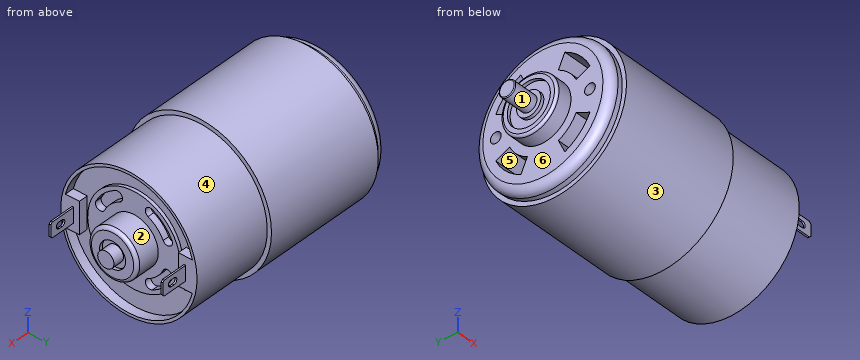
```python
from build123d import *

# Parameters (mm, degrees)
SKETCH1_W                      = 38
SKETCH1_H                      = 22.3
SKETCH2_R                      = 21
BOSS_EXTRUDE1_DEPTH            = 25
SKETCH3_W                      = 4.6
SKETCH3_H                      = 0.5
BOSS_EXTRUDE2_DEPTH            = 8.15
CUT_EXTRUDE1_DEPTH             = 40.8
SKETCH5_W                      = 4.6
SKETCH5_H                      = 0.5
BOSS_EXTRUDE3_DEPTH            = 8.15
CUT_EXTRUDE2_REACH             = 41.8
CUT_EXTRUDE3_DEPTH             = 2.8
SKETCH8_R                      = 14.25
BOSS_EXTRUDE4_DEPTH            = 1
CUT_EXTRUDE4_DEPTH             = 2
CUT_EXTRUDE5_DEPTH             = 2
CUT_EXTRUDE6_DEPTH             = 2
CUT_EXTRUDE7_DEPTH             = 2
SKETCH13_R                     = 21
BOSS_EXTRUDE5_DEPTH            = 4
CUT_EXTRUDE8_DEPTH             = 10
CUT_EXTRUDE9_DEPTH             = 10
CUT_EXTRUDE10_DEPTH            = 10
CUT_EXTRUDE11_DEPTH            = 10
SKETCH18_R                     = 7.5
BOSS_EXTRUDE6_DEPTH            = 7.6
F_8_0_8_DIAMETER_HOLE1_D       = 8
F_8_0_8_DIAMETER_HOLE1_DEPTH   = 1
SKETCH21_R                     = 8.65
BOSS_EXTRUDE7_DEPTH            = 5
M12_CLEARANCE_HOLE1_D          = 13.25
M12_CLEARANCE_HOLE1_DEPTH      = 1
SKETCH25_W                     = 3.4
SKETCH25_H                     = 2.5
F_2_5_2_5_DIAMETER_HOLE1_D     = 2.5
F_2_5_2_5_DIAMETER_HOLE1_DEPTH = 0.1
F_3_3_3_3_DIAMETER_HOLE1_D     = 3.3
F_3_3_3_3_DIAMETER_HOLE1_DEPTH = 11.5
F_3_3_3_3_DIAMETER_HOLE1_TIP   = 0.991420021
CHAMFER1_SIZE                  = 0.5
FILLET1_R                      = 0.25
FILLET2_R                      = 0.75
FILLET3_R                      = 1
FILLET4_R                      = 2.5


with BuildPart() as part:
    # Sketch1 → Revolve1 (revolve)
    with BuildSketch(Plane.XY):
        with Locations((23, 11.15)):
            Rectangle(SKETCH1_W, SKETCH1_H)
    revolve(axis=Axis((4, 0, 0), (1, 0, 0)))

    # Sketch2 → Boss-Extrude1 (add)
    with BuildSketch(Plane(origin=(42, 0, 0), x_dir=(0, 0, -1), z_dir=(1, 0, 0))):
        Circle(SKETCH2_R)
    extrude(amount=BOSS_EXTRUDE1_DEPTH)

    # Sketch3 → Boss-Extrude2 (add)
    with BuildSketch(Plane(origin=(67, 0, 0), x_dir=(0, 0, -1), z_dir=(1, 0, 0))):
        with Locations((0, 17.25)):
            Rectangle(SKETCH3_W, SKETCH3_H)
    extrude(amount=BOSS_EXTRUDE2_DEPTH)

    # Sketch4 → Cut-Extrude1 (cut, through all)
    with BuildSketch(Plane(origin=(0, 17.5, 0), x_dir=(-1, 0, 0), z_dir=(0, 1, 0))):
        with BuildLine():
            Line((-72.15, -1), (-71.15, -1))
            ThreePointArc((-71.15, -1), (-70.15, 0), (-71.15, 1))
            Line((-71.15, 1), (-72.15, 1))
            ThreePointArc((-72.15, 1), (-73.15, 0), (-72.15, -1))
        make_face()
    extrude(amount=-CUT_EXTRUDE1_DEPTH, mode=Mode.SUBTRACT)

    # Sketch5 → Boss-Extrude3 (add)
    with BuildSketch(Plane(origin=(67, 0, 0), x_dir=(0, 0, -1), z_dir=(1, 0, 0))):
        with Locations((0, -17.25)):
            Rectangle(SKETCH5_W, SKETCH5_H)
    extrude(amount=BOSS_EXTRUDE3_DEPTH)

    # Sketch6 → Cut-Extrude2 (cut, up to next)
    with BuildSketch(Plane.XZ.offset(17.5), mode=Mode.PRIVATE) as cut_extrude2_sk1:
        with BuildLine():
            Line((72.15, 1), (71.15, 1))
            ThreePointArc((71.15, 1), (70.15, 0), (71.15, -1))
            Line((71.15, -1), (72.15, -1))
            ThreePointArc((72.15, -1), (73.15, 0), (72.15, 1))
        make_face()
    cut_extrude2_tool1 = extrude(cut_extrude2_sk1.sketch, amount=-CUT_EXTRUDE2_REACH, mode=Mode.PRIVATE) & part.part
    add(cut_extrude2_tool1.solids().sort_by_distance((71.65, -17.5, 0))[0], mode=Mode.SUBTRACT)

    # Sketch7 → Cut-Extrude3 (cut)
    with BuildSketch(Plane(origin=(67, 0, 0), x_dir=(0, 0, -1), z_dir=(1, 0, 0))):
        with BuildLine():
            Line((4.875, 19.551390616), (4.875, 15.25))
            Line((4.875, 15.25), (-4.875, 15.25))
            Line((-4.875, 15.25), (-4.875, 19.551390616))
            ThreePointArc((-4.875, 19.551390616), (-20.15, 0), (-4.875, -19.551390616))
            Line((-4.875, -19.551390616), (-4.875, -15.25))
            Line((-4.875, -15.25), (4.875, -15.25))
            Line((4.875, -15.25), (4.875, -19.551390616))
            ThreePointArc((4.875, -19.551390616), (20.15, 0), (4.875, 19.551390616))
        make_face()
    extrude(amount=-CUT_EXTRUDE3_DEPTH, mode=Mode.SUBTRACT)

    # Sketch8 → Boss-Extrude4 (add)
    with BuildSketch(Plane(origin=(64.2, 0, 0), x_dir=(0, 0, -1), z_dir=(1, 0, 0))):
        Circle(SKETCH8_R)
    extrude(amount=BOSS_EXTRUDE4_DEPTH)

    # Sketch9 → Cut-Extrude4 (cut)
    with BuildSketch(Plane(origin=(65.2, 0, 0), x_dir=(0, 0, -1), z_dir=(1, 0, 0))):
        with BuildLine():
            ThreePointArc((-5.652173913, 11.706960752), (-9.192388155, 9.192388155), (-11.706960752, 5.652173913))
            ThreePointArc((-11.706960752, 5.652173913), (-11.008331502, 3.649196836), (-9.005354425, 4.347826087))
            ThreePointArc((-9.005354425, 4.347826087), (-7.071067812, 7.071067812), (-4.347826087, 9.005354425))
            ThreePointArc((-4.347826087, 9.005354425), (-3.649196836, 11.008331502), (-5.652173913, 11.706960752))
        make_face()
    extrude(amount=-CUT_EXTRUDE4_DEPTH, mode=Mode.SUBTRACT)

    # Sketch10 → Cut-Extrude5 (cut)
    with BuildSketch(Plane(origin=(65.2, 0, 0), x_dir=(0, 0, -1), z_dir=(1, 0, 0))):
        with BuildLine():
            ThreePointArc((11.706960752, 5.652173913), (9.192388155, 9.192388155), (5.652173913, 11.706960752))
            ThreePointArc((5.652173913, 11.706960752), (3.649196836, 11.008331502), (4.347826087, 9.005354425))
            ThreePointArc((4.347826087, 9.005354425), (7.071067812, 7.071067812), (9.005354425, 4.347826087))
            ThreePointArc((9.005354425, 4.347826087), (11.008331502, 3.649196836), (11.706960752, 5.652173913))
        make_face()
    extrude(amount=-CUT_EXTRUDE5_DEPTH, mode=Mode.SUBTRACT)

    # Sketch11 → Cut-Extrude6 (cut)
    with BuildSketch(Plane(origin=(65.2, 0, 0), x_dir=(0, 0, -1), z_dir=(1, 0, 0))):
        with BuildLine():
            ThreePointArc((5.652173913, -11.706960752), (9.192388155, -9.192388155), (11.706960752, -5.652173913))
            ThreePointArc((11.706960752, -5.652173913), (11.008331502, -3.649196836), (9.005354425, -4.347826087))
            ThreePointArc((9.005354425, -4.347826087), (7.071067812, -7.071067812), (4.347826087, -9.005354425))
            ThreePointArc((4.347826087, -9.005354425), (3.649196836, -11.008331502), (5.652173913, -11.706960752))
        make_face()
    extrude(amount=-CUT_EXTRUDE6_DEPTH, mode=Mode.SUBTRACT)

    # Sketch12 → Cut-Extrude7 (cut)
    with BuildSketch(Plane(origin=(65.2, 0, 0), x_dir=(0, 0, -1), z_dir=(1, 0, 0))):
        with BuildLine():
            ThreePointArc((-11.706960752, -5.652173913), (-9.192388155, -9.192388155), (-5.652173913, -11.706960752))
            ThreePointArc((-5.652173913, -11.706960752), (-3.649196836, -11.008331502), (-4.347826087, -9.005354425))
            ThreePointArc((-4.347826087, -9.005354425), (-7.071067812, -7.071067812), (-9.005354425, -4.347826087))
            ThreePointArc((-9.005354425, -4.347826087), (-11.008331502, -3.649196836), (-11.706960752, -5.652173913))
        make_face()
    extrude(amount=-CUT_EXTRUDE7_DEPTH, mode=Mode.SUBTRACT)

    # Sketch13 → Boss-Extrude5 (add)
    with BuildSketch(Plane.ZY.offset(-4)):
        Circle(SKETCH13_R)
    extrude(amount=BOSS_EXTRUDE5_DEPTH)

    # Sketch14 → Cut-Extrude8 (cut)
    with BuildSketch(Plane.ZY):
        with BuildLine():
            Line((6.761892188, 14.500924593), (4.775586358, 10.241277994))
            ThreePointArc((4.775586358, 10.241277994), (7.990306627, 7.990306627), (10.241277994, 4.775586358))
            Line((10.241277994, 4.775586358), (14.500924593, 6.761892188))
            ThreePointArc((14.500924593, 6.761892188), (11.313708499, 11.313708499), (6.761892188, 14.500924593))
        make_face()
    extrude(amount=-CUT_EXTRUDE8_DEPTH, mode=Mode.SUBTRACT)

    # Sketch15 → Cut-Extrude9 (cut)
    with BuildSketch(Plane.ZY):
        with BuildLine():
            Line((-6.761892188, -14.500924593), (-4.775586358, -10.241277994))
            ThreePointArc((-4.775586358, -10.241277994), (-7.990306627, -7.990306627), (-10.241277994, -4.775586358))
            Line((-10.241277994, -4.775586358), (-14.500924593, -6.761892188))
            ThreePointArc((-14.500924593, -6.761892188), (-11.313708499, -11.313708499), (-6.761892188, -14.500924593))
        make_face()
    extrude(amount=-CUT_EXTRUDE9_DEPTH, mode=Mode.SUBTRACT)

    # Sketch16 → Cut-Extrude10 (cut)
    with BuildSketch(Plane.ZY):
        with BuildLine():
            Line((-14.500924593, 6.761892188), (-10.241277994, 4.775586358))
            ThreePointArc((-10.241277994, 4.775586358), (-7.990306627, 7.990306627), (-4.775586358, 10.241277994))
            Line((-4.775586358, 10.241277994), (-6.761892188, 14.500924593))
            ThreePointArc((-6.761892188, 14.500924593), (-11.313708499, 11.313708499), (-14.500924593, 6.761892188))
        make_face()
    extrude(amount=-CUT_EXTRUDE10_DEPTH, mode=Mode.SUBTRACT)

    # Sketch17 → Cut-Extrude11 (cut)
    with BuildSketch(Plane.ZY):
        with BuildLine():
            Line((14.500924593, -6.761892188), (10.241277994, -4.775586358))
            ThreePointArc((10.241277994, -4.775586358), (7.990306627, -7.990306627), (4.775586358, -10.241277994))
            Line((4.775586358, -10.241277994), (6.761892188, -14.500924593))
            ThreePointArc((6.761892188, -14.500924593), (11.313708499, -11.313708499), (14.500924593, -6.761892188))
        make_face()
    extrude(amount=-CUT_EXTRUDE11_DEPTH, mode=Mode.SUBTRACT)

    # Sketch18 → Boss-Extrude6 (add)
    with BuildSketch(Plane(origin=(65.2, 0, 0), x_dir=(0, 0, -1), z_dir=(1, 0, 0))):
        Circle(SKETCH18_R)
    extrude(amount=BOSS_EXTRUDE6_DEPTH)

    # Ø8.0 (8) Diameter Hole1
    with Locations(Plane(origin=(72.8, 0, 0), x_dir=(0, 0, -1), z_dir=(1, 0, 0))):
        with Locations((0, 0)):
            Hole(F_8_0_8_DIAMETER_HOLE1_D / 2, depth=F_8_0_8_DIAMETER_HOLE1_DEPTH)

    # Sketch21 → Boss-Extrude7 (add)
    with BuildSketch(Plane.ZY):
        Circle(SKETCH21_R)
    extrude(amount=BOSS_EXTRUDE7_DEPTH)

    # M12 Clearance Hole1
    with Locations(Plane.ZY.offset(5)):
        with Locations((0, 0)):
            Hole(M12_CLEARANCE_HOLE1_D / 2, depth=M12_CLEARANCE_HOLE1_DEPTH)

    # Sketch24 → Revolve2 (revolve)
    with BuildSketch(Plane(origin=(0, 0, 0), x_dir=(-1, 0, 0), z_dir=(0, 0, -1))):
        Polygon((4, 3.75), (4, 0), (12.8, 0), (12.8, 2.5), (5, 2.5), (5, 3.75), align=None)
    revolve(axis=Axis((-4, 0, 0), (-1, 0, 0)))

    # Sketch25 → Revolve3 (revolve)
    with BuildSketch(Plane(origin=(0, 0, 0), x_dir=(-1, 0, 0), z_dir=(0, 0, -1))):
        with Locations((-73.5, 1.25)):
            Rectangle(SKETCH25_W, SKETCH25_H)
    revolve(axis=Axis((75.2, 0, 0), (-1, 0, 0)))

    # Ø2.5 (2.5) Diameter Hole1
    with Locations(Plane(origin=(64.2, 0, 0), x_dir=(0, 0, -1), z_dir=(1, 0, 0))):
        with Locations((6.5, 15)):
            Hole(F_2_5_2_5_DIAMETER_HOLE1_D / 2, depth=F_2_5_2_5_DIAMETER_HOLE1_DEPTH)

    # Ø3.3 (3.3) Diameter Hole1
    with Locations(Plane.ZY):
        with Locations((0, 14.5), (0, -14.5)):
            Hole(F_3_3_3_3_DIAMETER_HOLE1_D / 2, depth=F_3_3_3_3_DIAMETER_HOLE1_DEPTH)
            with Locations((0, 0, -(F_3_3_3_3_DIAMETER_HOLE1_DEPTH + F_3_3_3_3_DIAMETER_HOLE1_TIP / 2))):  # 118° drill point
                Cone(0, F_3_3_3_3_DIAMETER_HOLE1_D / 2, F_3_3_3_3_DIAMETER_HOLE1_TIP, mode=Mode.SUBTRACT)

    # Chamfer1
    chamfer1_edges = [part.edges().sort_by_distance(p)[0] for p in [
        (75.15, 17.25, -2.3),
        (75.15, 17.25, 2.3),
        (75.15, -17.25, -2.3),
        (75.15, -17.25, 2.3),
    ]]
    chamfer(chamfer1_edges, length=CHAMFER1_SIZE)

    # Fillet1
    fillet1_edges = [part.edges().sort_by_distance(p)[0] for p in [
        (-12.8, -2.5, 0),
    ]]
    fillet(fillet1_edges, radius=FILLET1_R)

    # Fillet2
    fillet2_edges = [part.edges().sort_by_distance(p)[0] for p in [
        (-5, 0, -8.65),
    ]]
    fillet(fillet2_edges, radius=FILLET2_R)

    # Fillet3
    fillet3_edges = [part.edges().sort_by_distance(p)[0] for p in [
        (72.8, 0, 7.5),
    ]]
    fillet(fillet3_edges, radius=FILLET3_R)

    # Fillet4
    fillet4_edges = [part.edges().sort_by_distance(p)[0] for p in [
        (0, 0, -21),
    ]]
    fillet(fillet4_edges, radius=FILLET4_R)


solid = part.part
```
The listing builds one solid part. Answer for the finished solid, in the listing's coordinates (mm). Face numbers are marked on the shaded views. A direction names the side the tool comes from. Coordinates: 2 decimals unless noted, no trailing zeros. Order: outer loops, then holes, each group sorted by start corner. A loop starts at its lowest first (then second) coordinate and runs counter-clockwise, first axis right, second up. Notation, with made-up numbers: M 74.25,43 L 127.25,43 A37 cw 127.25,80 Z; hole C 66,85 d4. An arc over 180 degrees is marked long. Answer as a JSON object with one key per item and string values. Group by question number.
1. Section A-A on x = 43 is taken. Write down the section's boundary in (y, z).
2. Straight lines are drawn through the part: line 1 (Y direction, x = 72, z = 0); line 2 (Z direction, x = 1, y = 12); line 3 (Y direction, x = -4.2, z = 0) (3 decimals). For each, find the intervals that lie inside material, in ascending order.
3. Flat-ended cylindrical pins translate along their axes: P1, Ø1.5, axis at y = -3, z = 14, coming from the +X side; P2, Ø4, axis at y = 15, z = -6.5, coming from the -X side; P3, Ø4, axis at y = 17, z = -13, coming from the +X side. Find the tip coordinate at first contact, or state that the pin passes through.
4. A tool of negligible diameter and unlimited length cuts with its end or side. For the marked faces 1, 2 and 3, from which of +Z, -Z, +X, -X, +Y, -Y can it reach the whole face along a straight path? Write none if from no direction.
5. Determine the mould class of the marked faces 4, 5 and 6 for opening direction Y: released by +Y, released by -Y, zero draft, split by the parting line, or undercut.
Values follow:
{
 "1": {"outline": "C 0,0 d42"},
 "2": {"line 1": "-7.48 to -4, -2.5 to 2.5, 4 to 7.48", "line 2": "-16.62 to -10.58, -5.6 to 5.6, 10.58 to 16.62", "line 3": "-8.65 to -6.625, -3.75 to 3.75, 6.625 to 8.65"},
 "3": {"P1": "x = 65.2", "P2": "x = 0", "P3": "x = 67"},
 "4": {"face 1": "-X", "face 2": "+X", "face 3": "+X, -X"},
 "5": {"face 4": "split by the parting line", "face 5": "undercut", "face 6": "zero draft"}
}
